Check sheet for the modelled part. Datum: model origin and axes. Units: mm. Face numbers are marked on the shaded views. A direction names the side the tool comes from. Coordinates: 2 decimals unless noted, no trailing zeros. Loops run counter-clockwise (first coordinate to the right, second up) from the corner with the lowest first, then second, coordinate; pieces in that order, holes last. Notation, with made-up numbers: (-13.75, 14) - (44.25, 14) arc R26 cw to (44.25, 37) - close; hole circle Ø5 at (-17.75, -27.75). An arc over 180 degrees is marked (long way). Answer as a JSON object with one key per item and string values. Group by question number.
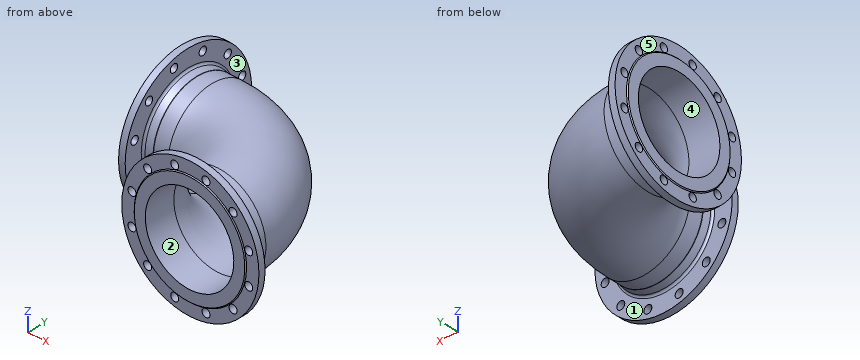
from build123d import *

# Parameters (mm, degrees)
CUT_EXTRUDE_1_REACH = 440.946
SKETCH_4_R          = 9
SKETCH_3_R          = 108
SKETCH_3_R_2        = 100


with BuildPart() as part:
    # Sketch 1 → Revolve 1 (revolve)
    with BuildSketch(Plane.XY, mode=Mode.PRIVATE) as revolve_1_sk:
        with BuildLine():
            Line((0, 350), (0, 375))
            Line((0, 375), (2, 377))
            Line((2, 377), (2, 405))
            Line((2, 405), (17, 405))
            Line((17, 405), (17, 365.72203777))
            ThreePointArc((17, 365.72203777), (18.169777784, 362.508099722), (21.131759112, 360.797999005))
            Line((21.131759112, 360.797999005), (36.569202429, 358.075961235))
            ThreePointArc((36.569202429, 358.075961235), (37.001664604, 358.01902651), (37.437443318, 358))
            Line((37.437443318, 358), (70, 358))
            Line((70, 358), (70, 350))
            Line((70, 350), (0, 350))
        make_face()
    revolve_1 = revolve(revolve_1_sk.sketch.rotate(Axis((0, 250, 0), (1, 0, 0)), 90), axis=Axis((0, 250, 0), (1, 0, 0)))

    # Sketch 4 → Cut-Extrude 1 (cut, up to next)
    with BuildSketch(Plane(origin=(2, 0, 0), x_dir=(0, 0, -1), z_dir=(1, 0, 0)), mode=Mode.PRIVATE) as cut_extrude_1_sk1:
        with Locations(Location((-35.328799656, 381.848875288, 0), (0, 0, 180))):
            Circle(SKETCH_4_R)
    cut_extrude_1_tool1 = extrude(cut_extrude_1_sk1.sketch, amount=CUT_EXTRUDE_1_REACH, mode=Mode.PRIVATE) & part.part
    # Sketch 4 → Cut-Extrude 1 (cut, up to next)
    with BuildSketch(Plane(origin=(2, 0, 0), x_dir=(0, 0, -1), z_dir=(1, 0, 0)), mode=Mode.PRIVATE) as cut_extrude_1_sk2:
        with Locations(Location((35.328799656, 381.848875288, 0), (0, 0, 180))):
            Circle(SKETCH_4_R)
    cut_extrude_1_tool2 = extrude(cut_extrude_1_sk2.sketch, amount=CUT_EXTRUDE_1_REACH, mode=Mode.PRIVATE) & part.part
    # Sketch 4 → Cut-Extrude 1 (cut, up to next)
    with BuildSketch(Plane(origin=(2, 0, 0), x_dir=(0, 0, -1), z_dir=(1, 0, 0)), mode=Mode.PRIVATE) as cut_extrude_1_sk3:
        with Locations(Location((96.520075632, 346.520075632, 0), (0, 0, 180))):
            Circle(SKETCH_4_R)
    cut_extrude_1_tool3 = extrude(cut_extrude_1_sk3.sketch, amount=CUT_EXTRUDE_1_REACH, mode=Mode.PRIVATE) & part.part
    # Sketch 4 → Cut-Extrude 1 (cut, up to next)
    with BuildSketch(Plane(origin=(2, 0, 0), x_dir=(0, 0, -1), z_dir=(1, 0, 0)), mode=Mode.PRIVATE) as cut_extrude_1_sk4:
        with Locations(Location((131.848875288, 285.328799656, 0), (0, 0, 180))):
            Circle(SKETCH_4_R)
    cut_extrude_1_tool4 = extrude(cut_extrude_1_sk4.sketch, amount=CUT_EXTRUDE_1_REACH, mode=Mode.PRIVATE) & part.part
    # Sketch 4 → Cut-Extrude 1 (cut, up to next)
    with BuildSketch(Plane(origin=(2, 0, 0), x_dir=(0, 0, -1), z_dir=(1, 0, 0)), mode=Mode.PRIVATE) as cut_extrude_1_sk5:
        with Locations(Location((131.848875288, 214.671200344, 0), (0, 0, 180))):
            Circle(SKETCH_4_R)
    cut_extrude_1_tool5 = extrude(cut_extrude_1_sk5.sketch, amount=CUT_EXTRUDE_1_REACH, mode=Mode.PRIVATE) & part.part
    # Sketch 4 → Cut-Extrude 1 (cut, up to next)
    with BuildSketch(Plane(origin=(2, 0, 0), x_dir=(0, 0, -1), z_dir=(1, 0, 0)), mode=Mode.PRIVATE) as cut_extrude_1_sk6:
        with Locations(Location((96.520075632, 153.479924368, 0), (0, 0, 180))):
            Circle(SKETCH_4_R)
    cut_extrude_1_tool6 = extrude(cut_extrude_1_sk6.sketch, amount=CUT_EXTRUDE_1_REACH, mode=Mode.PRIVATE) & part.part
    # Sketch 4 → Cut-Extrude 1 (cut, up to next)
    with BuildSketch(Plane(origin=(2, 0, 0), x_dir=(0, 0, -1), z_dir=(1, 0, 0)), mode=Mode.PRIVATE) as cut_extrude_1_sk7:
        with Locations(Location((35.328799656, 118.151124712, 0), (0, 0, 180))):
            Circle(SKETCH_4_R)
    cut_extrude_1_tool7 = extrude(cut_extrude_1_sk7.sketch, amount=CUT_EXTRUDE_1_REACH, mode=Mode.PRIVATE) & part.part
    # Sketch 4 → Cut-Extrude 1 (cut, up to next)
    with BuildSketch(Plane(origin=(2, 0, 0), x_dir=(0, 0, -1), z_dir=(1, 0, 0)), mode=Mode.PRIVATE) as cut_extrude_1_sk8:
        with Locations(Location((-35.328799656, 118.151124712, 0), (0, 0, 180))):
            Circle(SKETCH_4_R)
    cut_extrude_1_tool8 = extrude(cut_extrude_1_sk8.sketch, amount=CUT_EXTRUDE_1_REACH, mode=Mode.PRIVATE) & part.part
    # Sketch 4 → Cut-Extrude 1 (cut, up to next)
    with BuildSketch(Plane(origin=(2, 0, 0), x_dir=(0, 0, -1), z_dir=(1, 0, 0)), mode=Mode.PRIVATE) as cut_extrude_1_sk9:
        with Locations(Location((-96.520075632, 153.479924368, 0), (0, 0, 180))):
            Circle(SKETCH_4_R)
    cut_extrude_1_tool9 = extrude(cut_extrude_1_sk9.sketch, amount=CUT_EXTRUDE_1_REACH, mode=Mode.PRIVATE) & part.part
    # Sketch 4 → Cut-Extrude 1 (cut, up to next)
    with BuildSketch(Plane(origin=(2, 0, 0), x_dir=(0, 0, -1), z_dir=(1, 0, 0)), mode=Mode.PRIVATE) as cut_extrude_1_sk10:
        with Locations(Location((-131.848875288, 214.671200344, 0), (0, 0, 180))):
            Circle(SKETCH_4_R)
    cut_extrude_1_tool10 = extrude(cut_extrude_1_sk10.sketch, amount=CUT_EXTRUDE_1_REACH, mode=Mode.PRIVATE) & part.part
    # Sketch 4 → Cut-Extrude 1 (cut, up to next)
    with BuildSketch(Plane(origin=(2, 0, 0), x_dir=(0, 0, -1), z_dir=(1, 0, 0)), mode=Mode.PRIVATE) as cut_extrude_1_sk11:
        with Locations(Location((-131.848875288, 285.328799656, 0), (0, 0, 180))):
            Circle(SKETCH_4_R)
    cut_extrude_1_tool11 = extrude(cut_extrude_1_sk11.sketch, amount=CUT_EXTRUDE_1_REACH, mode=Mode.PRIVATE) & part.part
    # Sketch 4 → Cut-Extrude 1 (cut, up to next)
    with BuildSketch(Plane(origin=(2, 0, 0), x_dir=(0, 0, -1), z_dir=(1, 0, 0)), mode=Mode.PRIVATE) as cut_extrude_1_sk12:
        with Locations(Location((-96.520075632, 346.520075632, 0), (0, 0, 180))):
            Circle(SKETCH_4_R)
    cut_extrude_1_tool12 = extrude(cut_extrude_1_sk12.sketch, amount=CUT_EXTRUDE_1_REACH, mode=Mode.PRIVATE) & part.part
    cut_extrude_1_1 = cut_extrude_1_tool1.solids().sort_by_distance((2, 381.848875, 35.3288))[0]
    add(cut_extrude_1_1, mode=Mode.SUBTRACT)
    cut_extrude_1_2 = cut_extrude_1_tool2.solids().sort_by_distance((2, 381.848875, -35.3288))[0]
    add(cut_extrude_1_2, mode=Mode.SUBTRACT)
    cut_extrude_1_3 = cut_extrude_1_tool3.solids().sort_by_distance((2, 346.520076, -96.520076))[0]
    add(cut_extrude_1_3, mode=Mode.SUBTRACT)
    cut_extrude_1_4 = cut_extrude_1_tool4.solids().sort_by_distance((2, 285.3288, -131.848875))[0]
    add(cut_extrude_1_4, mode=Mode.SUBTRACT)
    cut_extrude_1_5 = cut_extrude_1_tool5.solids().sort_by_distance((2, 214.6712, -131.848875))[0]
    add(cut_extrude_1_5, mode=Mode.SUBTRACT)
    cut_extrude_1_6 = cut_extrude_1_tool6.solids().sort_by_distance((2, 153.479924, -96.520076))[0]
    add(cut_extrude_1_6, mode=Mode.SUBTRACT)
    cut_extrude_1_7 = cut_extrude_1_tool7.solids().sort_by_distance((2, 118.151125, -35.3288))[0]
    add(cut_extrude_1_7, mode=Mode.SUBTRACT)
    cut_extrude_1_8 = cut_extrude_1_tool8.solids().sort_by_distance((2, 118.151125, 35.3288))[0]
    add(cut_extrude_1_8, mode=Mode.SUBTRACT)
    cut_extrude_1_9 = cut_extrude_1_tool9.solids().sort_by_distance((2, 153.479924, 96.520076))[0]
    add(cut_extrude_1_9, mode=Mode.SUBTRACT)
    cut_extrude_1_10 = cut_extrude_1_tool10.solids().sort_by_distance((2, 214.6712, 131.848875))[0]
    add(cut_extrude_1_10, mode=Mode.SUBTRACT)
    cut_extrude_1_11 = cut_extrude_1_tool11.solids().sort_by_distance((2, 285.3288, 131.848875))[0]
    add(cut_extrude_1_11, mode=Mode.SUBTRACT)
    cut_extrude_1_12 = cut_extrude_1_tool12.solids().sort_by_distance((2, 346.520076, 96.520076))[0]
    add(cut_extrude_1_12, mode=Mode.SUBTRACT)
    cut_extrude_1 = cut_extrude_1_1 + cut_extrude_1_2 + cut_extrude_1_3 + cut_extrude_1_4 + cut_extrude_1_5 + cut_extrude_1_6 + cut_extrude_1_7 + cut_extrude_1_8 + cut_extrude_1_9 + cut_extrude_1_10 + cut_extrude_1_11 + cut_extrude_1_12  # Cut-Extrude 1 as one shape, for the pattern or mirror that repeats it

    # Sweep 1: sweep along a path in Sketch 2
    with BuildLine(Plane.XY) as sweep_1_path:
        ThreePointArc((70, 250), (197.279220614, 197.279220614), (250, 70))
    # Sketch 3 → Sweep 1 (sweep)
    with BuildSketch(Plane(origin=(70, 0, 0), x_dir=(0, 0, -1), z_dir=(1, 0, 0))):
        with Locations((0, 250)):
            Circle(SKETCH_3_R)
        with Locations((0, 250)):
            Circle(SKETCH_3_R_2, mode=Mode.SUBTRACT)
    sweep(path=sweep_1_path.line)

    # Mirror 1: Revolve 1, Cut-Extrude 1 across plane
    add(revolve_1.mirror(Plane(origin=(0, 0, 0), x_dir=(0, 0, 1), z_dir=(0.7071067811865475, -0.7071067811865477, 0))))
    add(cut_extrude_1.mirror(Plane(origin=(0, 0, 0), x_dir=(0, 0, 1), z_dir=(0.7071067811865475, -0.7071067811865477, 0))), mode=Mode.SUBTRACT)


solid = part.part
1. Gauge pin test, flat ends, axial feed: pin 1 (11 mm diameter, centred on x = 285.33, z = 131.85, fed in from +Y); pin 2 (4 mm diameter, centred on y = 312.5, z = -106.5, fed in from +X); pin 3 (23.5 mm diameter, centred on x = 153.48, z = 96.52, fed in from +Y); pin 4 (1.5 mm diameter, centred on x = 120, y = 212, fed in from +Z). Record the tip position at first contact, or that the pin passes through.
2. Release check for a two-part mould opening along X. For the marked faces 3, 4 and 5 record: released by +X, released by -X, zero draft, split by the parting line, or undercut.
3. Sectioned sample at A-A on y = 57.5. Record the cut outline in (x, z), plus the area to 3 significant figures.
4. Access from +Z, -Z, +X, -X, +Y, -Y to the whole of each face (thin tool, end or side, straight path). Record for the marked faces 1 and 2.
5. Material ranges on line 1 (X direction, y = 363, z = 84.5); line 2 (Z direction, x = 242.5, y = 266); line 3 (Z direction, x = 341, y = 88), recorded low to high.
Answers follow:
{
 "1": {"pin 1": "passes through", "pin 2": "stops at x = 17", "pin 3": "stops at y = 302.91", "pin 4": "stops at z = 104.12"},
 "2": {"face 3": "undercut", "face 4": "zero draft", "face 5": "released by -X"},
 "3": {"outline": "circle Ø216 at (250, 0); hole circle Ø200 at (250, 0)", "area": "5,230 mm^2"},
 "4": {"face 1": "none", "face 2": "-Y"},
 "5": {"line 1": "x = 2 to 17", "line 2": "z = -71.32 to -58.51, 58.51 to 71.32", "line 3": "z = -57.22 to -40.12, 40.12 to 57.22"}
}
